from build123d import *

# Parameters (mm, degrees)
SKETCH1_W           = 150
SKETCH1_H           = 100
BOSS_EXTRUDE1_DEPTH = 12.7
SKETCH2_W           = 13.263106726
SKETCH2_H           = 7.75
SKETCH2_R           = 2.75
CUT_EXTRUDE1_DEPTH  = 12.7
SKETCH3_R           = 2.75
CUT_EXTRUDE2_DEPTH  = 30
SKETCH5_W           = 7.5
SKETCH5_H           = 12.7
BOSS_EXTRUDE2_DEPTH = 10
SKETCH6_W           = 7.5
SKETCH6_H           = 12.7
BOSS_EXTRUDE3_DEPTH = 10
SKETCH4_R           = 1.25
CUT_EXTRUDE3_DEPTH  = 40


with BuildPart() as part:
    # Sketch1 → Boss-Extrude1 (new body)
    with BuildSketch(Plane(origin=(0, 0, 0), x_dir=(1, 0, 0), z_dir=(0, 1, 0))):
        with Locations((75, 50)):
            Rectangle(SKETCH1_W, SKETCH1_H)
    extrude(amount=BOSS_EXTRUDE1_DEPTH)

    # Sketch2 → Cut-Extrude1 (cut)
    with BuildSketch(Plane(origin=(0, 12.7, 0), x_dir=(1, 0, 0), z_dir=(0, 1, 0))):
        with BuildLine():
            ThreePointArc((81.631553363, 42.25), (84.265037623, 45.733962277), (85.2, 50))
            Line((85.2, 50), (81.631553363, 50))
            Line((81.631553363, 50), (81.631553363, 42.25))
        make_face()
        with BuildLine():
            Line((81.631553363, 50), (85.2, 50))
            ThreePointArc((85.2, 50), (84.265037623, 54.266037723), (81.631553363, 57.75))
            Line((81.631553363, 57.75), (81.631553363, 50))
        make_face()
        with BuildLine():
            Line((68.368446637, 42.25), (68.368446637, 50))
            Line((68.368446637, 50), (64.8, 50))
            ThreePointArc((64.8, 50), (65.734962377, 45.733962277), (68.368446637, 42.25))
        make_face()
        with BuildLine():
            Line((64.8, 50), (68.368446637, 50))
            Line((68.368446637, 50), (68.368446637, 57.75))
            ThreePointArc((68.368446637, 57.75), (65.734962377, 54.266037723), (64.8, 50))
        make_face()
        with Locations((75, 53.875)):
            Rectangle(SKETCH2_W, SKETCH2_H)
        with Locations((75, 46.125)):
            Rectangle(SKETCH2_W, SKETCH2_H)
        with Locations((10, 90)):
            Circle(SKETCH2_R)
        with Locations((140, 90)):
            Circle(SKETCH2_R)
        with Locations((140, 10)):
            Circle(SKETCH2_R)
        with Locations((10, 10)):
            Circle(SKETCH2_R)
    extrude(amount=-CUT_EXTRUDE1_DEPTH, mode=Mode.SUBTRACT)

    # Sketch3 → Cut-Extrude2 (cut)
    with BuildSketch(Plane(origin=(0, 12.7, 0), x_dir=(1, 0, 0), z_dir=(0, 1, 0))):
        with BuildLine():
            Line((133.5, 50), (146.5, 50))
            Line((146.5, 50), (146.5, 42.5))
            Line((146.5, 42.5), (146.5, 0))
            Line((146.5, 0), (150, 0))
            Line((150, 0), (150, 100))
            Line((150, 100), (0, 100))
            Line((0, 100), (0, 0))
            Line((0, 0), (3.5, 0))
            Line((3.5, 0), (3.5, 42.5))
            Line((3.5, 42.5), (3.5, 50))
            Line((3.5, 50), (16.5, 50))
            Line((16.5, 50), (59.8, 50))
            ThreePointArc((59.8, 50), (75, 65.2), (90.2, 50))
            Line((90.2, 50), (133.5, 50))
        make_face()
        with Locations((10, 90)):
            Circle(SKETCH3_R, mode=Mode.SUBTRACT)
        with Locations((140, 90)):
            Circle(SKETCH3_R, mode=Mode.SUBTRACT)
        with BuildLine():
            Line((85.2, 50), (90.2, 50))
            ThreePointArc((90.2, 50), (75, 65.2), (59.8, 50))
            Line((59.8, 50), (64.8, 50))
            ThreePointArc((64.8, 50), (65.734962377, 54.266037723), (68.368446637, 57.75))
            ThreePointArc((68.368446637, 57.75), (75, 60.2), (81.631553363, 57.75))
            ThreePointArc((81.631553363, 57.75), (84.265037623, 54.266037723), (85.2, 50))
        make_face()
        with BuildLine():
            Line((75, 50), (85.2, 50))
            ThreePointArc((85.2, 50), (84.265037623, 54.266037723), (81.631553363, 57.75))
            Line((81.631553363, 57.75), (68.368446637, 57.75))
            ThreePointArc((68.368446637, 57.75), (65.734962377, 54.266037723), (64.8, 50))
            Line((64.8, 50), (75, 50))
        make_face()
        with BuildLine():
            Line((133.5, 0), (133.5, 42.5))
            Line((133.5, 42.5), (88.220816919, 42.5))
            ThreePointArc((88.220816919, 42.5), (75, 34.8), (61.779183081, 42.5))
            Line((61.779183081, 42.5), (16.5, 42.5))
            Line((16.5, 42.5), (16.5, 0))
            Line((16.5, 0), (133.5, 0))
        make_face()
        with BuildLine():
            Line((75, 42.5), (75, 50))
            Line((75, 50), (64.8, 50))
            ThreePointArc((64.8, 50), (65.657812944, 45.90566965), (68.086968827, 42.5))
            Line((68.086968827, 42.5), (75, 42.5))
        make_face()
        with BuildLine():
            ThreePointArc((81.913031173, 42.5), (84.342187056, 45.90566965), (85.2, 50))
            Line((85.2, 50), (75, 50))
            Line((75, 50), (75, 42.5))
            Line((75, 42.5), (81.913031173, 42.5))
        make_face()
        with BuildLine():
            Line((68.368446637, 57.75), (81.631553363, 57.75))
            ThreePointArc((81.631553363, 57.75), (75, 60.2), (68.368446637, 57.75))
        make_face()
    extrude(amount=-CUT_EXTRUDE2_DEPTH, mode=Mode.SUBTRACT)

    # Sketch5 → Boss-Extrude2 (add)
    with BuildSketch(Plane(origin=(146.5, 0, 0), x_dir=(0, 0, -1), z_dir=(1, 0, 0))):
        with Locations((46.25, 6.35)):
            Rectangle(SKETCH5_W, SKETCH5_H)
    extrude(amount=BOSS_EXTRUDE2_DEPTH)

    # Sketch6 → Boss-Extrude3 (add)
    with BuildSketch(Plane.ZY.offset(-3.5)):
        with Locations((-46.25, 6.35)):
            Rectangle(SKETCH6_W, SKETCH6_H)
    extrude(amount=BOSS_EXTRUDE3_DEPTH)

    # Sketch4 → Cut-Extrude3 (cut)
    with BuildSketch(Plane(origin=(0, 0, -50), x_dir=(-1, 0, 0), z_dir=(0, 0, -1))):
        with Locations((-151.5, 6.35)):
            Circle(SKETCH4_R)
        with Locations((-93.2, 6.35)):
            Circle(SKETCH4_R)
        with Locations((-56.8, 6.35)):
            Circle(SKETCH4_R)
        with Locations((1.5, 6.35)):
            Circle(SKETCH4_R)
    extrude(amount=-CUT_EXTRUDE3_DEPTH, mode=Mode.SUBTRACT)


solid = part.part
Model file for the job. Use its own axes, mm. A direction names the side the tool comes from. Give positions to 0.01 mm unless a question says otherwise; leave off trailing zeros. Order: outer loops, then holes, each group sorted by start corner. A loop starts at its lowest first (then second) coordinate and runs counter-clockwise, first axis right, second up. Notation, with made-up numbers: M -26,59 L -13,59 A24 ccw -13,94 Z; hole C 5,59.25 d9. An arc over 180 degrees is marked long. Write item = value, one per line.
Q1. Cut at A-A, the plane z = -14.5. List the corners of the cut face in (x, y), then the cut area to 3 significant figures.
Derived:
outline = M 3.5,0 L 16.5,0 L 16.5,12.7 L 3.5,12.7 Z; M 133.5,0 L 146.5,0 L 146.5,12.7 L 133.5,12.7 Z
area = 330 mm2
Q2. Two-plate mould, pull along X, no slides. Class faces 5 (the flat face through (3.5, 6, -21)), 6 (the cylindrical face through (75.2, 6.4, -34.8)), 7 (the flat face through (156.5, 6, -46)): pulls with the +X half, pulls with the -X half, needs draft (parallel to the pull), parting line crosses it, or undercut.
Derived:
face_5 = pulls with the -X half
face_6 = undercut
face_7 = pulls with the +X half
Q3. Cut at D-D, the plane z = -46. List the corners of the cut face in (x, y).
Derived:
outline = M -6.5,0 L 65.62,0 L 65.62,12.7 L -6.5,12.7 Z; M 84.38,0 L 156.5,0 L 156.5,12.7 L 84.38,12.7 Z; hole C -1.5,6.35 d2.5; hole C 56.8,6.35 d2.5; hole C 93.2,6.35 d2.5; hole C 151.5,6.35 d2.5
Q4. Cut at B-B, the plane y = 11.25. List the corners of the cut face in (x, z), then the cut area to 3 significant figures.
Derived:
outline = M -6.5,-50 L 64.8,-50 A10.2 cw 68.37,-42.25 L 81.63,-42.25 A10.2 cw 85.2,-50 L 156.5,-50 L 156.5,-42.5 L 146.5,-42.5 L 146.5,0 L 133.5,0 L 133.5,-42.5 L 88.22,-42.5 A15.2 ccw 61.78,-42.5 L 16.5,-42.5 L 16.5,0 L 3.5,0 L 3.5,-42.5 L -6.5,-42.5 Z; hole C 10,-10 d5.5; hole C 140,-10 d5.5
area = 2,280 mm2
Q5. Drill centre lines: line 1 (X direction, y = 6.5, z = -10); line 2 (Y direction, x = 151.5, z = -45.5); line 3 (X direction, y = 12, z = -23). Where is each one in solid material? Low to high. Write a range as [from, to].
Derived:
line_1 = [3.5, 7.25], [12.75, 16.5], [133.5, 137.25], [142.75, 146.5]
line_2 = [0, 5.1], [7.6, 12.7]
line_3 = [3.5, 16.5], [133.5, 146.5]
Q6. Flat gauge pins, fed straight in: pin 1 (6.5 mm diameter, centred on x = 72, y = 6, fed in from -Z); pin 2 (3.5 mm diameter, centred on x = 10, z = -10, fed in from -Y); pin 3 (3 mm diameter, centred on x = 0, y = 7, fed in from +Z); pin 4 (4 mm diameter, centred on y = 4.5, z = -26.5, fed in from -X). Where does each tip first touch, or does it go through?
Derived:
pin_1 = -42.25
pin_2 = through
pin_3 = -42.5
pin_4 = 3.5
Q7. Cut at C-C, the plane x = 140. List the corners of the cut face in (y, z).
Derived:
outline = M 0,-50 L 12.7,-50 L 12.7,-12.75 L 0,-12.75 Z; M 0,-7.25 L 12.7,-7.25 L 12.7,0 L 0,0 Z
Q8. Tool access for faces 1 (the cylindrical face through (65.71, 6.44, -45.79)), 2 (the flat face through (146.5, 6, -22)), 3 (the flat face through (133.5, 6, -21)), 4 (the cylindrical face through (142.62, 6.44, -10.83)): list every direction of +Z, -Z, +X, -X, +Y, -Y with a clear straight run to the whole face (end or side of a thin tool).
Derived:
face_1 = -Z, +Y, -Y
face_2 = +Z, +X, +Y, -Y
face_3 = +Z, +Y, -Y
face_4 = +Y, -Y
